```python
from build123d import *

# Parameters (mm, degrees)
F0_W     = 42
F0_H     = 42
F1_DEPTH = 1800
F2_W     = 42
F2_H     = 42
F3_DEPTH = 1000
F4_W     = 42
F4_H     = 42
F5_DEPTH = 1800


with BuildPart() as f1:
    # F0 (on Top) → F1 (new body)
    with BuildSketch(Plane.XY):
        with Locations((21, -21)):
            Rectangle(F0_W, F0_H)
    extrude(amount=F1_DEPTH)

    # F2 (on face) → F3 (join)
    with BuildSketch(Plane.YZ.offset(42)):
        with Locations((-21, 1779)):
            Rectangle(F2_W, F2_H)
    extrude(amount=F3_DEPTH)

    # F4 (on face) → F5 (join)
    with BuildSketch(Plane.XY.offset(1800)):
        with Locations((1063, -21)):
            Rectangle(F4_W, F4_H)
    extrude(amount=-F5_DEPTH)


solid = f1.part
```
CAD build for the part. Positions are in the model's coordinates, mm. A direction names the side the tool comes from. Coordinates: 2 decimals unless noted, no trailing zeros. Order: outer loops, then holes, each group sorted by start corner. A loop starts at its lowest first (then second) coordinate and runs counter-clockwise, first axis right, second up. Notation, with made-up numbers: (71, -40) - (97, -40) arc R34 cw to (97, -4) - close; hole circle Ø1 at (9.5, 5). An arc over 180 degrees is marked (long way). Answer in a Markdown table with one row per item.
1. Slice it at A-A, the plane z = 149. List the corners of the cut face in (x, y).
Answer:
| item | result |
|---|---|
| outline | (0, -42) - (42, -42) - (42, 0) - (0, 0) - close; (1042, -42) - (1084, -42) - (1084, 0) - (1042, 0) - close |
2. 3-axis set-ups, long thin cutter, end or side, ignore diameter. For faces 4 (the face through (535, -21, 1758)), 5 (the face through (534, -21, 1800)): which of +Z, -Z, +X, -X, +Y, -Y reach the whole face in a straight line?
Answer:
| item | result |
|---|---|
| face 4 | -Z, +Y, -Y |
| face 5 | +Z, +X, -X, +Y, -Y |
3. Drill centre lines: L1, parallel to X at y = -12.5, z = 826; L2, parallel to Z at x = 208, y = -29. Where is each one in solid material? Low to high. Write a range as from..to.
Answer:
| item | result |
|---|---|
| L1 | 0..42, 1042..1084 |
| L2 | 1758..1800 |
4. Flat gauge pins, fed straight in: P1, Ø1.5, axis at x = 550, y = -34, coming from the -Z side; P2, Ø4, axis at y = -4, z = 1111.5, coming from the -X side. Where does each tip first touch, or does it go through?
Answer:
| item | result |
|---|---|
| P1 | z = 1758 |
| P2 | x = 0 |
5. Slice it at B-B, the plane y = -31.5. List the corners of the cut face in (x, z), then the cut area to 3 significant figures.
Answer:
| item | result |
|---|---|
| outline | (0, 0) - (42, 0) - (42, 1758) - (1042, 1758) - (1042, 0) - (1084, 0) - (1084, 1800) - (0, 1800) - close |
| area | 193,000 mm² |
6. Pull direction X, two halves, no side cores. Call faces 1 (the face through (42, -21, 867)), 2 (the face through (1063, -21, 0)), 3 (the face through (1084, -21, 913)): +X half, -X half, draft (parallel to the pull), parting line (faces both ways), or undercut.
Answer:
| item | result |
|---|---|
| face 1 | undercut |
| face 2 | draft |
| face 3 | +X half |
7. Slice it at C-C, the plane x = 874. List the corners of the cut face in (y, z).
Answer:
| item | result |
|---|---|
| outline | (-42, 1758) - (0, 1758) - (0, 1800) - (-42, 1800) - close |
